The model under review builds one solid part; all positions refer to its coordinate system, in mm. Face numbers are marked on the shaded views. A direction names the side the tool comes from. Give positions to 0.01 mm unless a question says otherwise; leave off trailing zeros. Order: outer loops, then holes, each group sorted by start corner. A loop starts at its lowest first (then second) coordinate and runs counter-clockwise, first axis right, second up. Notation, with made-up numbers: (39.25, 44) - (76.25, 44) arc R18 ccw to (76.25, 72) - close; hole circle Ø8 at (83, -3.5). An arc over 180 degrees is marked (long way). Answer as CSV lines item,"result". Start each with the question number.
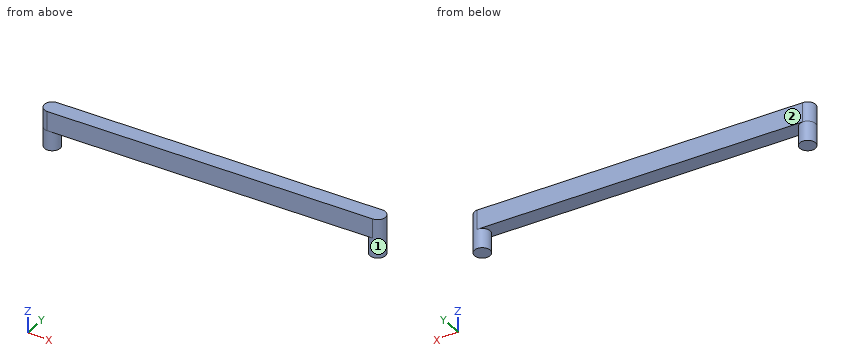
from build123d import *

# Parameters (mm, degrees)
SALIENTE_EXTRUIR1_DEPTH = 1.5
CROQUIS2_R              = 0.6
SALIENTE_EXTRUIR2_DEPTH = 1.5


with BuildPart() as part:
    # Croquis1 → Saliente-Extruir1 (new body)
    with BuildSketch(Plane.XY):
        with BuildLine():
            Line((0, 0.6), (24.2, 1.9))
            ThreePointArc((24.2, 1.9), (24.8, 1.3), (24.2, 0.7))
            Line((24.2, 0.7), (0, -0.6))
            ThreePointArc((0, -0.6), (-0.6, 0), (0, 0.6))
        make_face()
    extrude(amount=SALIENTE_EXTRUIR1_DEPTH)

    # Croquis2 → Saliente-Extruir2 (add)
    with BuildSketch(Plane(origin=(0, 0, 0), x_dir=(-1, 0, 0), z_dir=(0, 0, -1))):
        with Locations((-24.2, 1.3)):
            Circle(CROQUIS2_R)
        Circle(CROQUIS2_R)
    extrude(amount=SALIENTE_EXTRUIR2_DEPTH)


solid = part.part
Item 1: Machinability: for the marked faces 1 and 2, which of the approach directions +Z, -Z, +X, -X, +Y, -Y give a long, thin tool a straight path to every point of the face, cutting with its end or side? Answer none if there is none.
Item 2: Take a section at B-B on y = 0. Write out the cut boundary in (x, z), and give its area (3 significant figures).
Item 3: Clearance check with a flat-ended pin moving along its axis: pin 1 (0.7 mm diameter, centred on x = 9, y = 1, fed in from -Z). State where the tip first meets the part, or that it passes through.
Item 4: Take a section at A-A on z = -0.25. Write out the cut boundary in (x, y), and give its area (3 significant figures).
Item 5: For line 1 along Z through (x, y) = (18.5, 1.45); line 2 along X through (y, z) = (0.05, -0.75); line 3 along Y through (x, z) = (4.75, 1.35), list the stretches that pass through material, from the lowest coordinate up.
Item 6: Take a section at C-C on x = 19.5. Write out the cut boundary in (y, z), and give its area (3 significant figures).
Data:
1,face 1,"-Z"
1,face 2,"+Z, -Z, -X, +Y"
2,outline,"(-0.6, -1.5) - (0.6, -1.5) - (0.6, 0) - (11.17, 0) - (11.17, 1.5) - (-0.6, 1.5) - close"
2,area,"19.5 mm^2"
3,pin 1,"stops at z = 0"
4,outline,"circle Ø1.2 at (0, 0); circle Ø1.2 at (24.2, 1.3)"
4,area,"2.26 mm^2"
5,line 1,"z = 0 to 1.5"
5,line 2,"x = -0.6 to 0.6"
5,line 3,"y = -0.34 to 0.86"
6,outline,"(0.45, 0) - (1.65, 0) - (1.65, 1.5) - (0.45, 1.5) - close"
6,area,"1.80 mm^2"
